```python
from build123d import *

# Parameters (mm, degrees)
F0_R     = 1.5
F1_DEPTH = 36
F2_R     = 30
F3_R     = 5


with BuildPart() as f1:
    # F0 (on Top) → F1 (new body)
    with BuildSketch(Plane.XY):
        with BuildLine():
            Line((3.7082439195, 81), (0, 81))
            Line((0, 81), (0, 78))
            Line((0, 78), (1.8262379212, 78))
            ThreePointArc((1.8262379212, 78), (2.8946339641, 79.4200818425), (3.7082439195, 81))
        make_face()
        with BuildLine():
            Line((1.8262379212, 78), (0, 78))
            Line((0, 78), (0, 76.3831560302))
            ThreePointArc((0, 76.3831560302), (0.9602269984, 77.1383691176), (1.8262379212, 78))
        make_face()
        with BuildLine():
            Line((15.7082439195, 81), (3.7082439195, 81))
            ThreePointArc((3.7082439195, 81), (2.8946339641, 79.4200818425), (1.8262379212, 78))
            ThreePointArc((1.8262379212, 78), (0.9602269984, 77.1383691176), (0, 76.3831560302))
            ThreePointArc((0, 76.3831560302), (8.9608411477, 74.9261020604), (15.7082439195, 81))
        make_face()
        with BuildLine():
            ThreePointArc((7.5, 78), (6, 76.5), (4.5, 78))
            ThreePointArc((4.5, 78), (6, 79.5), (7.5, 78))
        make_face(mode=Mode.SUBTRACT)
        Polygon((35.2081528017, 85), (0, 85), (0, 81), (3.7082439195, 81), (15.7082439195, 81), (23.6789969548, 81), (33.5512985522, 81), (40.5320699577, 74.0192285946), (74.0192285946, 40.5320699577), (81, 33.5512985522), (81, 23.6789969548), (81, -23.6789969548), (81, -33.5512985522), (74.0192285946, -40.5320699577), (40.5320699577, -74.0192285946), (33.5512985522, -81), (35.2081528017, -85), (85, -35.2081528017), (85, 35.2081528017), align=None)
        with BuildLine():
            Line((33.5512985522, 81), (23.6789969548, 81))
            ThreePointArc((23.6789969548, 81), (30.5381379027, 73.7255866944), (40.5320699577, 74.0192285946))
            Line((40.5320699577, 74.0192285946), (33.5512985522, 81))
        make_face()
        with Locations((32.1454083187, 77.6058807309)):
            Circle(F0_R, mode=Mode.SUBTRACT)
        with BuildLine():
            ThreePointArc((74.0192285946, 40.5320699577), (73.7255866944, 30.5381379027), (81, 23.6789969548))
            Line((81, 23.6789969548), (81, 33.5512985522))
            Line((81, 33.5512985522), (74.0192285946, 40.5320699577))
        make_face()
        with Locations((77.6058807309, 32.1454083187)):
            Circle(F0_R, mode=Mode.SUBTRACT)
        with BuildLine():
            ThreePointArc((81, -23.6789969548), (73.7255866944, -30.5381379027), (74.0192285946, -40.5320699577))
            Line((74.0192285946, -40.5320699577), (81, -33.5512985522))
            Line((81, -33.5512985522), (81, -23.6789969548))
        make_face()
        with Locations((77.6058807309, -32.1454083187)):
            Circle(F0_R, mode=Mode.SUBTRACT)
        with BuildLine():
            Line((23.6789969548, -81), (33.5512985522, -81))
            Line((33.5512985522, -81), (40.5320699577, -74.0192285946))
            ThreePointArc((40.5320699577, -74.0192285946), (30.5381379027, -73.7255866944), (23.6789969548, -81))
        make_face()
        with Locations((32.1454083187, -77.6058807309)):
            Circle(F0_R, mode=Mode.SUBTRACT)
        Polygon((0, -81), (0, -85), (35.2081528017, -85), (33.5512985522, -81), (23.6789969548, -81), (15.7082439195, -81), (3.7082439195, -81), align=None)
        with BuildLine():
            ThreePointArc((0, -76.3831560302), (2.1863327454, -78.4247466831), (3.7082439195, -81))
            Line((3.7082439195, -81), (15.7082439195, -81))
            ThreePointArc((15.7082439195, -81), (8.9608411477, -74.9261020604), (0, -76.3831560302))
        make_face()
        with Locations((6, -78)):
            Circle(F0_R, mode=Mode.SUBTRACT)
        with BuildLine():
            Line((0, -76.3831560302), (0, -81))
            Line((0, -81), (3.7082439195, -81))
            ThreePointArc((3.7082439195, -81), (2.1863327454, -78.4247466831), (0, -76.3831560302))
        make_face()
    extrude(amount=F1_DEPTH)

    # F2
    f2_edges = [f1.edges().sort_by_distance(p)[0] for p in [
        (85, -35.208153, 18),
        (85, 35.208153, 18),
        (35.208153, 85, 18),
        (35.208153, -85, 18),
    ]]
    fillet(f2_edges, radius=F2_R)

    # F3
    f3_edges = [f1.edges().sort_by_distance(p)[0] for p in [
        (23.678997, 81, 18),
        (15.708244, 81, 18),
        (74.019229, 40.53207, 18),
        (81, 23.678997, 18),
        (81, -23.678997, 18),
        (74.019229, -40.53207, 18),
        (40.53207, -74.019229, 18),
        (15.708244, -81, 18),
        (23.678997, -81, 18),
    ]]
    fillet(f3_edges, radius=F3_R)


solid = f1.part
```
Check sheet for the modelled part. Datum: model origin and axes. Units: mm. A direction names the side the tool comes from. Give positions to 0.01 mm unless a question says otherwise; leave off trailing zeros. Write each loop counter-clockwise with the first axis right and the second up, starting at its lowest first coordinate (ties: lowest second). Pieces come first, ordered by that corner, then holes. Notation, with made-up numbers: (38.25, 26.25) - (79.25, 26.25) arc R35 cw to (79.25, 64.25) - close; hole circle Ø6 at (-12.5, 74.25). An arc over 180 degrees is marked (long way). Answer as a JSON object with one key per item and string values. Group by question number.
1) Depth check by flat-ended pin: P1, Ø5, axis at x = 77.61, y = -32.15, coming from the +Z side; P2, Ø1.5, axis at y = -47.5, z = 20.5, coming from the -X side; P3, Ø8, axis at x = 30, z = 13.5, coming from the -Y side; P4, Ø1, axis at x = 72, z = 10, coming from the +Y side. Enter the tip coordinate at first touch or a pass-through.
2) Release check for a two-part mould opening along Y. For faces 1 (the face through (78.99, 31.57, 17.75)), 2 (the face through (0, 81, 18)), 3 (the face through (82.78, 34.11, 18.25)) record: pulls with the +Y half, pulls with the -Y half, needs draft (parallel to the pull), parting line crosses it, or undercut.
3) Sectioned sample at D-D (z = 9.5). Give the number of separate pieces and of enclosed holes in the cut face, then the cut area to 3 significant figures.
4) Sectioned sample at A-A (x = 12). Record the cut outline in (y, z), then the cut area to 3 significant figures.
5) Access from +Z, -Z, +X, -X, +Y, -Y to the whole of each face (thin tool, end or side, straight path). Record for faces 4 (the face through (30.6, -73.7, 17.7)), 5 (the face through (85, 0, 18)).
6) Thickness scan on probe 1 along Y at (x, z) = (6, 16); probe 2 along Y at (x, z) = (33.5, 15.5); probe 3 along X at (y, z) = (78, 18.5). Record the ranges inside material, lowest first. Write a range as from..to.
7) Sectioned sample at B-B (y = 9.5). Record the cut outline in (x, z), then the cut area to 3 significant figures.
8) Sectioned sample at C-C (x = 28). Record the cut outline in (y, z), then the cut area to 3 significant figures.
Geometry results:
{
 "1": {"P1": "stops at z = 36", "P2": "stops at x = 66.3", "P3": "stops at y = -84.83", "P4": "stops at y = 48.71"},
 "2": {"face 1": "undercut", "face 2": "needs draft", "face 3": "pulls with the +Y half"},
 "3": {"separate pieces": "1", "enclosed holes": "6", "area": "1,500 mm^2"},
 "4": {"outline": "(-85, 0) - (-76.38, 0) - (-76.38, 36) - (-85, 36) - close; (76.38, 0) - (85, 0) - (85, 36) - (76.38, 36) - close", "area": "620 mm^2"},
 "5": {"face 4": "+Z, -Z", "face 5": "+Z, -Z, +X, +Y, -Y"},
 "6": {"probe 1": "y = -85..-79.5, -76.5..-74.5, 74.5..76.5, 79.5..85", "probe 2": "y = -83.02..-78.25, -76.96..-72.92, 72.92..76.96, 78.25..83.02", "probe 3": "x = 0..4.5, 7.5..13.83, 25.21..30.7, 33.59..42.04"},
 "7": {"outline": "(81, 0) - (85, 0) - (85, 36) - (81, 36) - close", "area": "144 mm^2"},
 "8": {"outline": "(-84.54, 0) - (-75.15, 0) - (-75.15, 36) - (-84.54, 36) - close; (75.15, 0) - (84.54, 0) - (84.54, 36) - (75.15, 36) - close", "area": "676 mm^2"}
}
